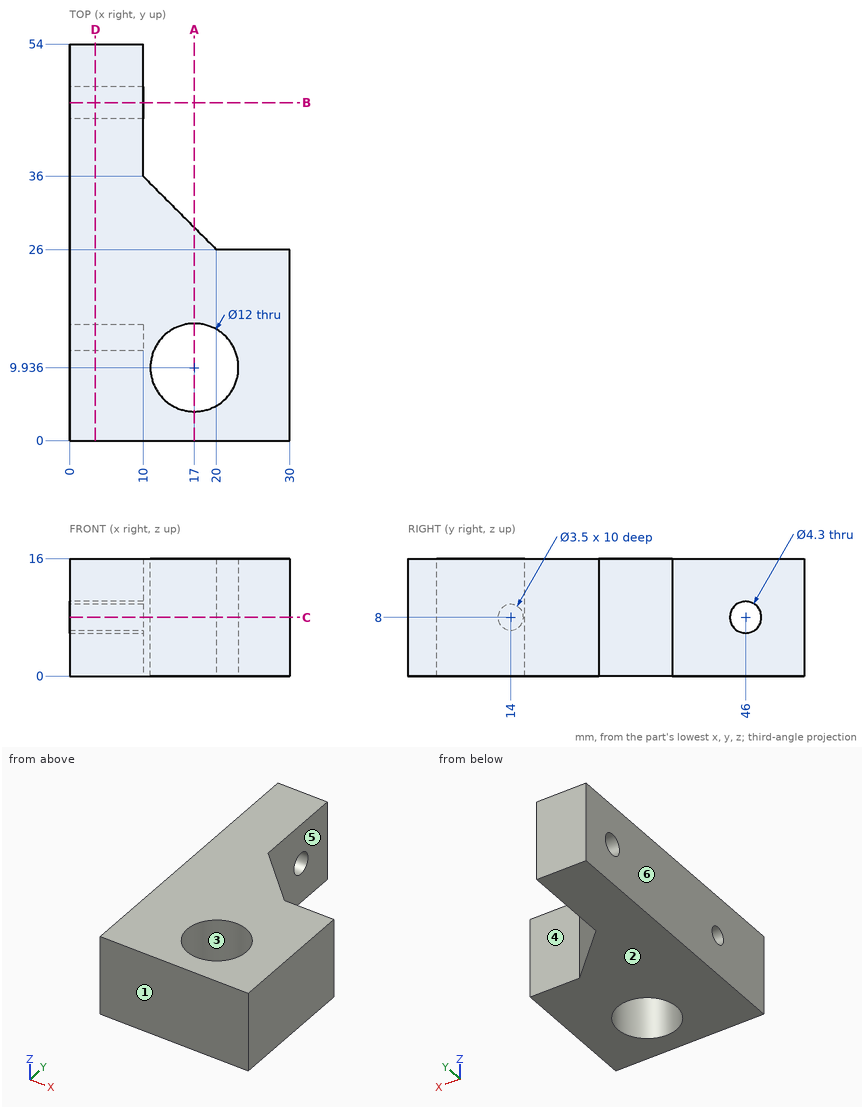
For this review, use the dimensioned drawing (mm, ordinates from the lowest corner) and the shaded views. A direction names the side the tool comes from. Give positions to 0.01 mm unless a question says otherwise; leave off trailing zeros. Order: outer loops, then holes, each group sorted by start corner. A loop starts at its lowest first (then second) coordinate and runs counter-clockwise, first axis right, second up. Notation, with made-up numbers: M -26,-25 L 18,-25 A28 ccw 18,4 Z; hole C -31.75,77.5 d3. An arc over 180 degrees is marked long. One line per question, with ' | ' between items. Start each with the question number.
1) Mouldability with a two-part tool opening along Y and no side actions: class the marked faces 1, 2, 3 and 4 as pulls with the +Y half, pulls with the -Y half, needs draft (parallel to the pull), parting line crosses it, or undercut.
2) Consider section C-C, the plane z = 8. Give the boundary of the cut face in (x, y), then the cut area to 3 significant figures.
3) Clearance check with flat-ended pins moving along their axes: P1, Ø5, axis at x = 19, z = 6.5, coming from the +Y side; P2, Ø3, axis at y = 45.5, z = 3.5, coming from the +X side; P3, Ø15.5, axis at x = 17, y = 9.94, coming from the +Z side; P4, Ø5, axis at x = 25, z = 6, coming from the +Y side. State where each tip first meets the part, or that it passes through.
4) Consider section A-A, the plane x = 17. Give the boundary of the cut face in (y, z), then the cut area to 3 significant figures.
5) For the marked faces 5 and 6, list the 3-axis set-ups (+Z, -Z, +X, -X, +Y, -Y) from which the entire face can be reached by the end or side of a thin tool; tool diameter is ignored.
6) Wall thickness on L1, parallel to Y at x = 7.5, z = 8; L2, parallel to Y at x = 1.5, z = 8.75 (1 decimal); L3, parallel to X at y = 44, z = 3: over which ranges is each line inside the solid? List them lowest first. Write a range as from..to.
7) Consider section D-D, the plane x = 3.5. Give the boundary of the cut face in (y, z), then the cut area to 3 significant figures.
8) Consider section B-B, the plane y = 46. Give the boundary of the cut face in (x, z), then the cut area to 3 significant figures.
Found:
1) face 1: pulls with the -Y half | face 2: needs draft | face 3: undercut | face 4: pulls with the +Y half
2) outline: M 0,0 L 30,0 L 30,26 L 20,26 L 10,36 L 10,43.85 L 0,43.85 L 0,15.75 L 10,15.75 L 10,12.25 L 0,12.25 Z; M 0,48.15 L 10,48.15 L 10,54 L 0,54 Z; hole C 17,9.94 d12 | area: 919 mm²
3) P1: stops at y = 29.5 | P2: stops at x = 10 | P3: stops at z = 16 | P4: stops at y = 26
4) outline: M 0,0 L 3.94,0 L 3.94,16 L 0,16 Z; M 15.94,0 L 29,0 L 29,16 L 15.94,16 Z | area: 272 mm²
5) face 5: +Z, -Z, +X, +Y | face 6: +Z, -Z, -X, +Y, -Y
6) L1: y = 0..12.25, 15.75..43.85, 48.15..54 | L2: y = 0..12.4, 15.6..44, 48..54 | L3: x = 0..10
7) outline: M 0,0 L 54,0 L 54,16 L 0,16 Z; hole C 14,8 d3.5; hole C 46,8 d4.3 | area: 840 mm²
8) outline: M 0,0 L 10,0 L 10,5.85 L 0,5.85 Z; M 0,10.15 L 10,10.15 L 10,16 L 0,16 Z | area: 117 mm²
